```python
from build123d import *

# Parameters (mm, degrees)
SKETCH_1_R      = 2
SKETCH_1_W      = 8.7
SKETCH_1_H      = 18
EXTRUDE_1_DEPTH = 5
FILLET_1_R      = 2


with BuildPart() as part:
    # 草图1 → 凸台-拉伸1 (new body)
    # profile 1 of 3: a face of its own
    with BuildSketch(Plane.XY):
        with BuildLine():
            Line((39, 40), (-39, 40))
            Line((-39, 40), (-39, 0))
            Line((-39, 0), (-30.3, 0))
            ThreePointArc((-30.3, 0), (0, 30.3), (30.3, 0))
            Line((30.3, 0), (39, 0))
            Line((39, 0), (39, 40))
        make_face()
        with Locations((-34.65, 10)):
            Circle(SKETCH_1_R, mode=Mode.SUBTRACT)
        with Locations((34.65, 10)):
            Circle(SKETCH_1_R, mode=Mode.SUBTRACT)
    # profile 2 of 3: a face of its own
    with BuildSketch(Plane.XY):
        with Locations((-34.65, -9)):
            Rectangle(SKETCH_1_W, SKETCH_1_H)
        with Locations((-34.65, -10)):
            Circle(SKETCH_1_R, mode=Mode.SUBTRACT)
    # profile 3 of 3: a face of its own
    with BuildSketch(Plane.XY):
        with Locations((34.65, -9)):
            Rectangle(SKETCH_1_W, SKETCH_1_H)
        with Locations((34.65, -10)):
            Circle(SKETCH_1_R, mode=Mode.SUBTRACT)
    extrude(amount=EXTRUDE_1_DEPTH)

    # 圆角1
    fillet_1_edges = [part.edges().sort_by_distance(p)[0] for p in [
        (-30.3, -18, 2.5),
        (-39, -18, 2.5),
        (-39, 40, 2.5),
        (39, 40, 2.5),
        (39, -18, 2.5),
        (30.3, -18, 2.5),
    ]]
    fillet(fillet_1_edges, radius=FILLET_1_R)


solid = part.part
```
The listing builds one solid part. Answer for the finished solid, in the listing's coordinates (mm). A direction names the side the tool comes from. Round coordinates to 2 decimals unless told otherwise and drop trailing zeros. Order: outer loops, then holes, each group sorted by start corner. A loop starts at its lowest first (then second) coordinate and runs counter-clockwise, first axis right, second up. Notation, with made-up numbers: (25.5, -34.5) -> (79.5, -34.5) arc R19 cw to (79.5, -13.5) -> close; hole circle Ø5 at (-24, -37.75). An arc over 180 degrees is marked (long way). Answer as CSV lines item,"result".
Q1. A cutting plane is placed at C-C on z = 2.35. Determine the outline of the cut face in (x, y).
Computed values:
outline,"(-39, -16) arc R2 ccw to (-37, -18) -> (-32.3, -18) arc R2 ccw to (-30.3, -16) -> (-30.3, 0) arc R30.3 cw to (30.3, 0) -> (30.3, -16) arc R2 ccw to (32.3, -18) -> (37, -18) arc R2 ccw to (39, -16) -> (39, 38) arc R2 ccw to (37, 40) -> (-37, 40) arc R2 ccw to (-39, 38) -> close; hole circle Ø4 at (-34.65, -10); hole circle Ø4 at (-34.65, 10); hole circle Ø4 at (34.65, -10); hole circle Ø4 at (34.65, 10)"
Q2. A cutting plane is placed at B-B on x = 34.65. Determine the outline of the cut face in (y, z), plus the area to 3 significant figures.
Computed values:
outline,"(-18, 0) -> (-12, 0) -> (-12, 5) -> (-18, 5) -> close; (-8, 0) -> (8, 0) -> (8, 5) -> (-8, 5) -> close; (12, 0) -> (40, 0) -> (40, 5) -> (12, 5) -> close"
area,"250 mm^2"
Q3. For a pull along Y with two mould halves and no side action, classify faces 3 (the cylindrical face through (38.43, -17.4, 2.54)), 4 (the cylindrical face through (-32.742, 10.601, 2.465)), 5 (the flat face through (1, 40, 2)), 6 (the flat face through (-39, 11, 2)) as +Y half, -Y half, draft (parallel to the pull), parting line (faces both ways), or undercut.
Computed values:
face 3,"-Y half"
face 4,"undercut"
face 5,"+Y half"
face 6,"draft"
Q4. Consider line 1 (Y direction, x = 34.65, z = 3.3); line 2 (X direction, y = -3.5, z = 3.8); line 3 (X direction, y = -11.5, z = 1.5). Determine where each line is inside the solid, lowest interval first. Write a range as from..to.
Computed values:
line 1,"y = -18..-12, -8..8, 12..40"
line 2,"x = -39..-30.3, 30.3..39"
line 3,"x = -39..-35.97, -33.33..-30.3, 30.3..33.33, 35.97..39"
Q5. A cutting plane is placed at D-D on y = 9. Determine the outline of the cut face in (x, z), plus the area to 3 significant figures.
Computed values:
outline,"(-39, 0) -> (-36.38, 0) -> (-36.38, 5) -> (-39, 5) -> close; (-32.92, 0) -> (-28.93, 0) -> (-28.93, 5) -> (-32.92, 5) -> close; (28.93, 0) -> (32.92, 0) -> (32.92, 5) -> (28.93, 5) -> close; (36.38, 0) -> (39, 0) -> (39, 5) -> (36.38, 5) -> close"
area,"66.0 mm^2"
Q6. Which of the six approach directions +Z, -Z, +X, -X, +Y, -Y give full straight-line access (tool end or side, diameter ignored) to faces 1 (the cylindrical face through (-32.742, -9.399, 2.465)), 2 (the flat face through (30.3, -8, 2))?
Computed values:
face 1,"+Z, -Z"
face 2,"+Z, -Z, -Y"
Q7. Given pin 1 (1.5 mm diameter, centred on x = 25, z = 4.5, fed in from -Y); pin 2 (2 mm diameter, centred on x = 13, z = 4.5, fed in from -Y); pin 3 (3 mm diameter, centred on x = -23.5, z = 3.5, fed in from -Y); pin 4 (3.5 mm diameter, centred on x = -34.65, y = 10, fed in from -Z), each flat-ended and moving along its own axis, determine where each tip first touches the part or whether it passes through.
Computed values:
pin 1,"stops at y = 15.97"
pin 2,"stops at y = 26.87"
pin 3,"stops at y = 17.12"
pin 4,"passes through"
Q8. A cutting plane is placed at A-A on y = -3.5. Determine the outline of the cut face in (x, z), plus the area to 3 significant figures.
Computed values:
outline,"(-39, 0) -> (-30.3, 0) -> (-30.3, 5) -> (-39, 5) -> close; (30.3, 0) -> (39, 0) -> (39, 5) -> (30.3, 5) -> close"
area,"87.0 mm^2"
